Autodesk Inventor part; units mm, degrees
ref_plane "YZ Plane" through (0, 0, 0) normal (1, 0, 0) x (0, 1, 0)
ref_plane "XZ Plane" through (0, 0, 0) normal (0, 1, 0) x (-1, 0, 0)
ref_plane "XY Plane" through (0, 0, 0) normal (0, 0, 1) x (1, 0, 0)
sketch "Sketch1" plane through (0, 0, 0) normal (0, 0, 1) x (1, 0, 0)
  line L0 (-12.1708, 16.0073) -> (13.2292, 16.0073)
  line L1 (13.2292, 16.0073) -> (13.2292, -34.7927)
  line L2 (13.2292, -34.7927) -> (-12.1708, -34.7927)
  line L3 (-12.1708, -34.7927) -> (-12.1708, 16.0073)
  line L4 (11.9592, 14.7373) -> (-10.9008, 14.7373)
  line L5 (-10.9008, 14.7373) -> (-10.9008, -33.5227)
  line L6 (-10.9008, -33.5227) -> (11.9592, -33.5227)
  line L7 (11.9592, -33.5227) -> (11.9592, 14.7373)
  point P0 (0, 0)
  dimension "d0" = 25.4
  dimension "d1" = 50.8
  dimension "d2" = 1.27
extrude "Extrusion1" add sketch "Sketch1" along normal blind 609.6
sketch "Sketch2" plane through (-12.1708, 16.0073, 0) normal (0, 1, 0) x (1, 0, 0)
  circle A0 centre (12.7, -12.7) radius 1.7272
  line L0 (25.4, 0) -> (0, 0)
  line L1 (0, 0) -> (0, -609.6)
  point P0 (12.1708, 0)
  dimension "d5" = 3.4544
  dimension "d6" = 12.7
  dimension "d7" = 12.7
extrude "Extrusion2" cut sketch "Sketch2" against normal through all
pattern_linear "Rectangular Pattern1" count 24 spacing 25.4 along (0, 0, 1) of "Extrusion2"
equation "\"d3\" = d13"
equation "\"d13\" = 609.6"
properties part number "VerseFrame 24in"
Geometry: final body of the model. Coordinates: model frame, mm. A direction names the side the tool comes from. Round coordinates to 2 decimals unless told otherwise and drop trailing zeros. Loops run counter-clockwise (first coordinate to the right, second up) from the corner with the lowest first, then second, coordinate; pieces in that order, holes last.
Q1. Section A-A on x = -5.5. Return loops of the section in (y, z), plus the area to 3 significant figures.
Q2. Section C-C on z = 538.5. Return loops of the section in (x, y).
Q3. Material intervals for L1, parallel to Y at x = 1, z = 558; L2, parallel to X at y = -19, z = 349.5; L3, parallel to X at y = 15, z = 292, sorted ascending.
Q4. Access query for faces 4 (the flat face through (1, -34.793, 301)), 5 (the flat face through (11.959, -10, 301)). Directions: +Z, -Z, +X, -X, +Y, -Y. A direction counts if a zero-diameter tool reaches every point of the face in a straight line with its end or side. Return the directions, or none.
Q5. Pull-direction query (X, two-part tool) for faces 1 (the flat face through (13.229, -9, 301)), 2 (the flat face through (-12.171, -10, 301)), 3 (the flat face through (0, -33.523, 301)); classes: released by +X, released by -X, zero draft, split by the parting line, or undercut.
Q6. Section B-B on y = -20. Return loops of the section in (x, z), plus the area to 3 significant figures.
Evaluation:
1. outline: (-34.79, 0) - (-33.52, 0) - (-33.52, 609.6) - (-34.79, 609.6) - close; (14.74, 0) - (16.01, 0) - (16.01, 609.6) - (14.74, 609.6) - close
1. area: 1,550 mm2
2. outline: (-12.17, -34.79) - (13.23, -34.79) - (13.23, 16.01) - (-12.17, 16.01) - close; hole (-10.9, -33.52) - (11.96, -33.52) - (11.96, 14.74) - (-10.9, 14.74) - close
3. L1: y = -34.79 to -33.52, 14.74 to 16.01
3. L2: x = -12.17 to -10.9, 11.96 to 13.23
3. L3: x = -12.17 to -1.2, 2.25 to 13.23
4. face 4: +Z, -Z, +X, -X, -Y
4. face 5: +Z, -Z
5. face 1: released by +X
5. face 2: released by -X
5. face 3: undercut
6. outline: (-12.17, 0) - (-10.9, 0) - (-10.9, 609.6) - (-12.17, 609.6) - close; (11.96, 0) - (13.23, 0) - (13.23, 609.6) - (11.96, 609.6) - close
6. area: 1,550 mm2
